Part model, mm, in its own coordinate system. A direction names the side the tool comes from. Coordinates: 2 decimals unless noted, no trailing zeros. Write each loop counter-clockwise with the first axis right and the second up, starting at its lowest first coordinate (ties: lowest second). Pieces come first, ordered by that corner, then holes. Notation, with made-up numbers: (38.5, -37) - (53.5, -37) arc R29 ccw to (53.5, -15) - close; hole circle Ø7 at (-10.75, 64.5). An arc over 180 degrees is marked (long way). Use one line per item in the form item = value. Start each with the question number.
from build123d import *

# Parameters (mm, degrees)
F1_DEPTH     = 20
F3_DEPTH     = 80
F5_DEPTH     = 20
F6_T4_DEPTH  = 1530.1801622923
F6_S5_R      = 100
F6_T6_DEPTH  = 767
F6_T10_DEPTH = 1530.1801622923
F6_S11_R     = 100
F6_T12_DEPTH = 767
F6_T16_DEPTH = 1530.1801622923
F6_S17_R     = 100
F6_T18_DEPTH = 767
F6_T22_DEPTH = 1530.1801622923
F6_S23_R     = 100
F6_T24_DEPTH = 767


# Not quite as in the source:
# - a fillet or chamfer that OpenCascade refuses, or shapes differently, is made with other operations: its cross-section is extruded or revolved along the edge and cut away or added


with BuildPart() as f1:
    # F0 (on Top) → F1 (new body)
    with BuildSketch(Plane.XY):
        with BuildLine():
            Line((1600, -53), (1600, 0))
            Line((1600, 0), (1600, 53))
            Line((1600, 53), (91.7986928012, 53))
            Line((91.7986928012, 53), (86.6025403784, 50))
            ThreePointArc((86.6025403784, 50), (100, 0), (86.6025403784, -50))
            Line((86.6025403784, -50), (91.7986928012, -53))
            Line((91.7986928012, -53), (1600, -53))
        make_face()
    extrude(amount=F1_DEPTH)

    # F2 (on face) → F3 (join)
    with BuildSketch(Plane.XY.offset(20)):
        with BuildLine():
            ThreePointArc((99.8198377077, 6), (100, 0), (99.8198377077, -6))
            Line((99.8198377077, -6), (1600, -6))
            Line((1600, -6), (1600, 6))
            Line((1600, 6), (99.8198377077, 6))
        make_face()
    extrude(amount=F3_DEPTH)

    # F4 (on face) → F5 (join)
    with BuildSketch(Plane.XY.offset(100)):
        with BuildLine():
            ThreePointArc((86.6025403784, 50), (100, 0), (86.6025403784, -50))
            Line((86.6025403784, -50), (91.7986928012, -53))
            Line((91.7986928012, -53), (1600, -53))
            Line((1600, -53), (1600, 53))
            Line((1600, 53), (91.7986928012, 53))
            Line((91.7986928012, 53), (86.6025403784, 50))
        make_face()
    extrude(amount=F5_DEPTH)

    # F6: fillet of radius 12 on 4 edges, made by hand


with BuildPart() as f6_tool2:
    # F6_s3 → F6_t4 (new body)
    with BuildSketch(Plane.YZ.offset(1600)):
        with BuildLine():
            ThreePointArc((6, 32), (9.5147186258, 23.5147186258), (18, 20))
            Line((18, 20), (6, 20))
            Line((6, 20), (6, 32))
        make_face()
    extrude(amount=-F6_T4_DEPTH)

    # F6_s5 → F6_t6 (cut, symmetric)
    with BuildSketch(Plane.XY.offset(26)):
        Circle(F6_S5_R)
    extrude(amount=F6_T6_DEPTH, both=True, mode=Mode.SUBTRACT)


with BuildPart() as f1_1:
    add(f1.part)

    # F6_t1: union F6_tool2
    add(f6_tool2.part)


with BuildPart() as f6_tool8:
    # F6_s9 → F6_t10 (new body)
    with BuildSketch(Plane.YZ.offset(69.8198377077)):
        with BuildLine():
            ThreePointArc((-6, 32), (-9.5147186258, 23.5147186258), (-18, 20))
            Line((-18, 20), (-6, 20))
            Line((-6, 20), (-6, 32))
        make_face()
    extrude(amount=F6_T10_DEPTH)

    # F6_s11 → F6_t12 (cut, symmetric)
    with BuildSketch(Plane.XY.offset(26)):
        Circle(F6_S11_R)
    extrude(amount=F6_T12_DEPTH, both=True, mode=Mode.SUBTRACT)


with BuildPart() as f1_2:
    add(f1_1.part)

    # F6_t7: union F6_tool8
    add(f6_tool8.part)


with BuildPart() as f6_tool14:
    # F6_s15 → F6_t16 (new body)
    with BuildSketch(Plane.YZ.offset(1600)):
        with BuildLine():
            ThreePointArc((18, 100), (9.5147186258, 96.4852813742), (6, 88))
            Line((6, 88), (6, 100))
            Line((6, 100), (18, 100))
        make_face()
    extrude(amount=-F6_T16_DEPTH)

    # F6_s17 → F6_t18 (cut, symmetric)
    with BuildSketch(Plane.XY.offset(94)):
        Circle(F6_S17_R)
    extrude(amount=F6_T18_DEPTH, both=True, mode=Mode.SUBTRACT)


with BuildPart() as f1_3:
    add(f1_2.part)

    # F6_t13: union F6_tool14
    add(f6_tool14.part)


with BuildPart() as f6_tool20:
    # F6_s21 → F6_t22 (new body)
    with BuildSketch(Plane.YZ.offset(69.8198377077)):
        with BuildLine():
            ThreePointArc((-18, 100), (-9.5147186258, 96.4852813742), (-6, 88))
            Line((-6, 88), (-6, 100))
            Line((-6, 100), (-18, 100))
        make_face()
    extrude(amount=F6_T22_DEPTH)

    # F6_s23 → F6_t24 (cut, symmetric)
    with BuildSketch(Plane.XY.offset(94)):
        Circle(F6_S23_R)
    extrude(amount=F6_T24_DEPTH, both=True, mode=Mode.SUBTRACT)


with BuildPart() as f1_4:
    add(f1_3.part)

    # F6_t19: union F6_tool20
    add(f6_tool20.part)


solid = f1_4.part
Q1. Pin check, flat tips, straight feed: P1, Ø17, axis at x = 902.5, z = 60, coming from the +Y side; P2, Ø5, axis at x = 733, z = 26, coming from the +Y side; P3, Ø2, axis at x = 361.5, z = 65.5, coming from the -Y side. Stop position of each tip, or through.
Q2. Mould opens along Z. For faces 4 (the flat face through (833, 1, 120)), 5 (the flat face through (833, -35, 20)), 6 (the flat face through (1600, -1, 74)) say: released by +Z, released by -Z, zero draft, split by the parting line, or undercut.
Q3. Drill centre lines: probe 1 along Z at (x, y) = (1445, -45); probe 2 along Z at (x, y) = (1295.5, 16); probe 3 along Y at (x, z) = (1326, 34). Where is each one in solid material? Low to high.
Q4. Which spindle directions (+Z, -Z, +X, -X, +Y, -Y) get a long thin tool onto all of the face, cutting with end or side? Do faces 1 (the flat face through (839, -6, 60)), 2 (the cylindrical face through (99.997, -0.733, 74.173)), 3 (the flat face through (833, 36, 100)). Say none if no direction does.
Q5. Slice it at C-C (z = 54). List the corners of the cut face in (x, y), plus the area to 3 significant figures.
Q6. Slice it at A-A (x = 1168.5). List the corners of the cut face in (y, z), plus the area to 3 significant figures.
Q7. Slice it at B-B (y = -32.5). List the corners of the cut face in (x, z), plus the area to 3 significant figures.
Solution:
q1.P1 = 6
q1.P2 = 9.53
q1.P3 = -6
q2.face_4 = released by +Z
q2.face_5 = undercut
q2.face_6 = zero draft
q3.probe_1 = 0 to 20, 100 to 120
q3.probe_2 = 0 to 20.17, 99.83 to 120
q3.probe_3 = -6 to 6
q4.face_1 = +X, -X, -Y
q4.face_2 = +Z, -Z, -X
q4.face_3 = +X, -X, +Y
q5.outline = (99.82, -6) - (1600, -6) - (1600, 6) - (99.82, 6) arc R100 cw to start
q5.area = 18,000 mm2
q6.outline = (-53, 0) - (53, 0) - (53, 20) - (18, 20) arc R12 cw to (6, 32) - (6, 88) arc R12 cw to (18, 100) - (53, 100) - (53, 120) - (-53, 120) - (-53, 100) - (-18, 100) arc R12 cw to (-6, 88) - (-6, 32) arc R12 cw to (-18, 20) - (-53, 20) - close
q6.area = 5,320 mm2
q7.outline = (94.57, 0) - (1600, 0) - (1600, 20) - (94.57, 20) - close; (94.57, 100) - (1600, 100) - (1600, 120) - (94.57, 120) - close
q7.area = 60,200 mm2
